Here's the drawing with two shaded views (mm, measured from the low corner). I have some questions. Give positions to 0.01 mm unless a question says otherwise; leave off trailing zeros. Loops run counter-clockwise (first coordinate to the right, second up) from the corner with the lowest first, then second, coordinate; pieces in that order, holes last. Notation, with made-up numbers: (21.5, 60.5) -> (60.5, 60.5) arc R8 cw to (60.5, 70.5) -> close; hole circle Ø6 at (-32, 73). An arc over 180 degrees is marked (long way). Put each result on its own line as item: value.
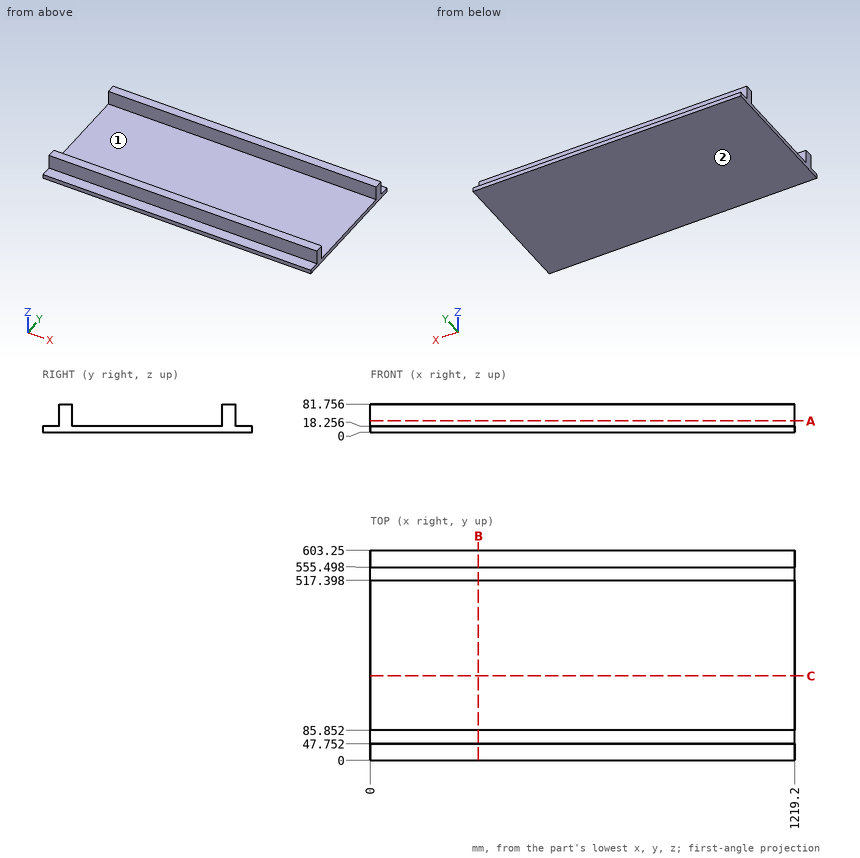
1. If we section it at B-B (x = 310.5): List the corners of the cut face in (y, z) for me.
Recorded:
outline: (0, 0) -> (603.25, 0) -> (603.25, 18.26) -> (555.5, 18.26) -> (555.5, 81.76) -> (517.4, 81.76) -> (517.4, 18.26) -> (85.85, 18.26) -> (85.85, 81.76) -> (47.75, 81.76) -> (47.75, 18.26) -> (0, 18.26) -> close
2. Thinking about a two-plate mould opening in Y: for the marked faces 1 and 2, which applies, pulls with the +Y half, pulls with the -Y half, needs draft (parallel to the pull), parting line crosses it, or undercut?
Recorded:
face 1: undercut
face 2: needs draft
3. If we section it at A-A (z = 33.5): List the corners of the cut face in (x, y) for me, then the cut area to 3 significant figures.
Recorded:
outline: (0, 47.75) -> (1219.2, 47.75) -> (1219.2, 85.85) -> (0, 85.85) -> close; (0, 517.4) -> (1219.2, 517.4) -> (1219.2, 555.5) -> (0, 555.5) -> close
area: 92,900 mm^2
4. I need wall thicknesses on line 1 (Y direction, x = 1154.5, z = 29); line 2 (Z direction, x = 179, y = 357.5). Which ranges of each line are inside material? Lowest first, please.
Recorded:
line 1: y = 47.75 to 85.85, 517.4 to 555.5
line 2: z = 0 to 18.26
5. If we section it at C-C (y = 242.5): List the corners of the cut face in (x, z) for me.
Recorded:
outline: (0, 0) -> (1219.2, 0) -> (1219.2, 18.26) -> (0, 18.26) -> close
6. I'm going to push flat-ended pins straight in: pin 1 (14.5 mm diameter, centred on x = 848.5, y = 568, fed in from +Z); pin 2 (12 mm diameter, centred on x = 1036.5, z = 57, fed in from -Y). Where does each tip first touch, or does it pass through?
Recorded:
pin 1: stops at z = 18.26
pin 2: stops at y = 47.75
